Here's how the part is built. I have some questions about the finished solid (model axes, mm). A direction names the side the tool comes from. Round coordinates to 2 decimals unless told otherwise and drop trailing zeros. Order: outer loops, then holes, each group sorted by start corner. A loop starts at its lowest first (then second) coordinate and runs counter-clockwise, first axis right, second up. Notation, with made-up numbers: (45.25, 80.25) -> (54.25, 80.25) arc R23 ccw to (54.25, 111.25) -> close; hole circle Ø5 at (42.25, 60.25). An arc over 180 degrees is marked (long way). Use a Markdown table: item, result. Add a question column.
(1) I want a section at B-B, the plane y = 6.35. Please give me the cut outline in (x, z).
(2) If I drill on probe 1 along Y at (x, z) = (6.35, 0.75) (3 decimals); probe 2 along Y at (x, z) = (25, 0.45) (3 decimals); probe 3 along X at (y, z) = (30.5, 1) (3 decimals), over which ranges is the centre line in solid material (lowest first)?
(3) I want a section at A-A, the plane x = 24. Please give me the cut outline in (y, z) (1 decimal), then the cut area to 3 significant figures.
(4) I want a section at C-C, the plane y = 28. Please give me the cut outline in (x, z) (1 decimal).
(5) I'm going to push a flat-ended pin straight in: P1, Ø8, axis at x = 24.5, y = 37.5, coming from the -Z side. Where does the tip first touch, or does it pass through?
(6) Thinking about a two-plate mould opening in Y: for faces 1 (the face through (0.905, 91.12, 0.783)), 2 (the face through (31.28, 87.86, 0.78)), 3 (the face through (0, 47, 1)), which applies, pulls with the +Y half, pulls with the -Y half, needs draft (parallel to the pull), parting line crosses it, or undercut?
(7) On a 3-axis mill with a long thin cutter (end or side, diameter ignored), from which of +Z, -Z, +X, -X, +Y, -Y can I reach the whole of each face in a straight line? I mean faces 4 (the face through (19, 15.875, 1)), 5 (the face through (6, 47, 1.588)). Say none if no direction works.
(8) I want a section at D-D, the plane x = 6.35. Please give me the cut outline in (y, z) (1 decimal), then the cut area to 3 significant figures.
Autodesk Inventor part; units mm, degrees
ref_plane "YZ Plane" through (0, 0, 0) normal (1, 0, 0) x (0, 1, 0)
ref_plane "XZ Plane" through (0, 0, 0) normal (0, 1, 0) x (-1, 0, 0)
ref_plane "XY Plane" through (0, 0, 0) normal (0, 0, 1) x (1, 0, 0)
sketch "Sketch1" plane through (0, 0, 0) normal (0, 0, 1) x (1, 0, 0)
  line L0 (3.175, 0) -> (34.925, 0)
  line L1 (38.1, 3.175) -> (38.1, 88.9)
  line L2 (34.925, 92.075) -> (3.175, 92.075)
  line L3 (0, 88.9) -> (0, 3.175)
  circle A0 centre (6.35, 85.725) radius 2.1844
  circle A1 centre (31.75, 85.725) radius 2.1844
  circle A2 centre (31.75, 6.35) radius 2.1844
  circle A3 centre (6.35, 6.35) radius 2.1844
  arc A4 (3.175, 92.075) -> (0, 88.9) centre (3.175, 88.9) ccw
  arc A5 (38.1, 88.9) -> (34.925, 92.075) centre (34.925, 88.9) ccw
  arc A6 (34.925, 0) -> (38.1, 3.175) centre (34.925, 3.175) ccw
  arc A7 (0, 3.175) -> (3.175, 0) centre (3.175, 3.175) ccw
  line L4 (9.525, 60.325) -> (28.575, 60.325)
  line L5 (28.575, 60.325) -> (28.575, 15.875)
  line L6 (28.575, 15.875) -> (9.525, 15.875)
  line L7 (9.525, 15.875) -> (9.525, 60.325)
  point P0 (0, 0)
  point P1 (38.1, 92.075)
  point P2 (38.1, 0)
  point P3 (0, 92.075)
  dimension "d0" = 38.1
  dimension "d1" = 92.075
  dimension "d2" = 4.3688
  dimension "d3" = 4.3688
  dimension "d4" = 4.3688
  dimension "d5" = 4.3688
  dimension "d6" = 0
  dimension "d7" = 25.4
  dimension "d8" = 0
  dimension "d9" = 79.375
  dimension "d10" = 0
  dimension "d11" = 79.375
  dimension "d12" = 6.35
  dimension "d13" = 6.35
  dimension "d14" = 3.175
  dimension "d16" = 25.4
  dimension "d17" = 9.525
  dimension "d18" = 9.525
  dimension "d19" = 9.525
extrude "Extrusion1" add sketch "Sketch1" along normal blind 1.5875
properties part number "odompoly"
Taken from the geometry:
| question | item | result |
|---|---|---|
| 1 | outline | (0, 0) -> (4.17, 0) -> (4.17, 1.59) -> (0, 1.59) -> close; (8.53, 0) -> (29.57, 0) -> (29.57, 1.59) -> (8.53, 1.59) -> close; (33.93, 0) -> (38.1, 0) -> (38.1, 1.59) -> (33.93, 1.59) -> close |
| 2 | probe 1 | y = 0 to 4.166, 8.534 to 83.541, 87.909 to 92.075 |
| 2 | probe 2 | y = 0 to 15.875, 60.325 to 92.075 |
| 2 | probe 3 | x = 0 to 9.525, 28.575 to 38.1 |
| 3 | outline | (0, 0) -> (15.9, 0) -> (15.9, 1.6) -> (0, 1.6) -> close; (60.3, 0) -> (92.1, 0) -> (92.1, 1.6) -> (60.3, 1.6) -> close |
| 3 | area | 75.6 mm2 |
| 4 | outline | (0, 0) -> (9.5, 0) -> (9.5, 1.6) -> (0, 1.6) -> close; (28.6, 0) -> (38.1, 0) -> (38.1, 1.6) -> (28.6, 1.6) -> close |
| 5 | P1 | passes through |
| 6 | face 1 | pulls with the +Y half |
| 6 | face 2 | undercut |
| 6 | face 3 | needs draft |
| 7 | face 4 | +Z, -Z |
| 7 | face 5 | +Z, +X, -X, +Y, -Y |
| 8 | outline | (0, 0) -> (4.2, 0) -> (4.2, 1.6) -> (0, 1.6) -> close; (8.5, 0) -> (83.5, 0) -> (83.5, 1.6) -> (8.5, 1.6) -> close; (87.9, 0) -> (92.1, 0) -> (92.1, 1.6) -> (87.9, 1.6) -> close |
| 8 | area | 132 mm2 |
